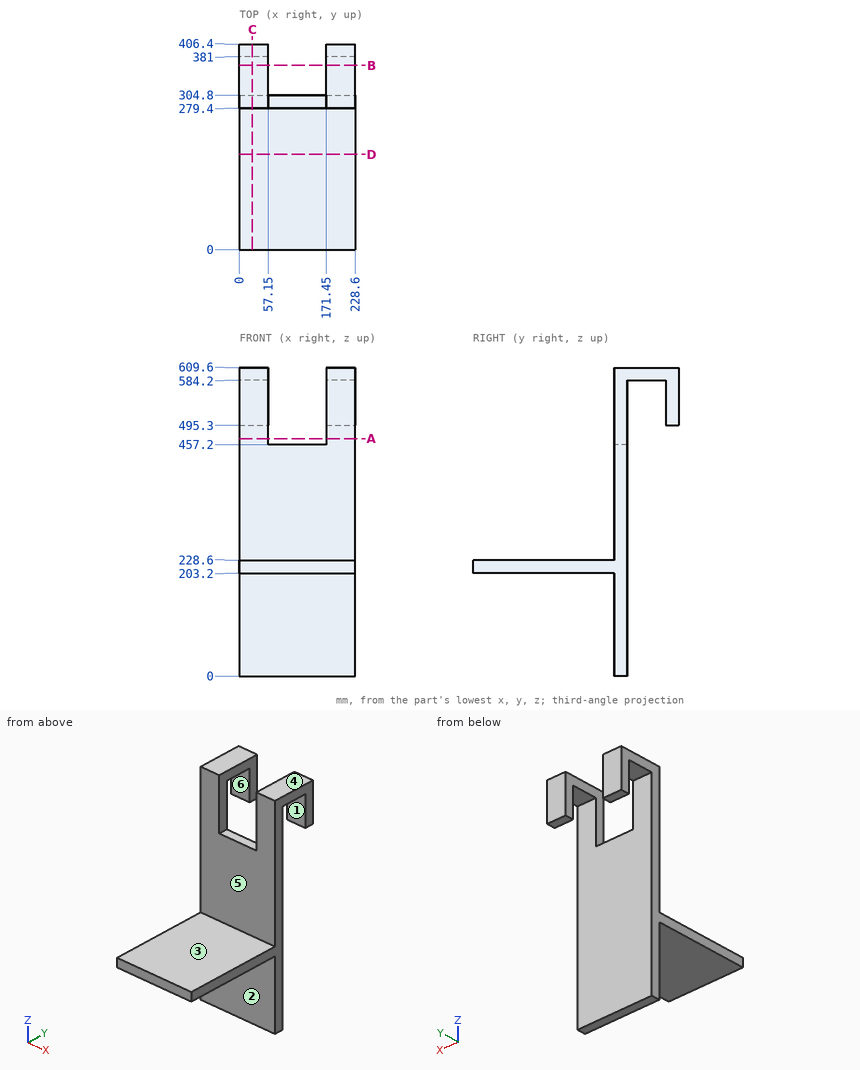
Geometry: see drawing. Coordinates: mm, zero at the bounding-box minimum. A direction names the side the tool comes from. Give positions to 0.01 mm unless a question says otherwise; leave off trailing zeros. Loops run counter-clockwise (first coordinate to the right, second up) from the corner with the lowest first, then second, coordinate; pieces in that order, holes last. Notation, with made-up numbers: (29.5, 61) - (46.5, 61) arc R19 cw to (46.5, 74) - close; hole circle Ø1 at (-11, 69). An arc over 180 degrees is marked (long way). Use CSV: the item, a comma, the result in double quotes. Start each with the question number.
1. Section B-B (y = 364). Output: boundary loops of the cut face in (x, z).
2. Reachability of the marked faces 1, 2 and 3 from +Z, -Z, +X, -X, +Y, -Y: full face, straight path, thin tool, end or side. Return the list, or none.
3. Pin query (flat end, axial travel): pin 1 (2 mm diameter, centred on x = 182, z = 534, fed in from -Y); pin 2 (7.5 mm diameter, centred on x = 91, y = 297, fed in from +Z); pin 3 (1 mm diameter, centred on x = 53, y = 174.5, fed in from -Z). Return the tip coordinate at first contact, or that it passes through.
4. Section C-C (x = 25.5). Output: boundary loops of the cut face in (y, z), then the cut area to 3 significant figures.
5. Section D-D (y = 188). Output: boundary loops of the cut face in (x, z), then the cut area to 3 significant figures.
6. Section A-A (z = 469). Output: boundary loops of the cut face in (x, y), then the cut area to 3 significant figures.
7. Draft query along Y for the marked faces 4, 5 and 6. Return one class per face: +Y half, -Y half, draft (parallel to the pull), parting line (faces both ways), or undercut.
8. Ray query, L1, parallel to X at y = 304.5, z = 529.5; L2, parallel to Y at x = 173, z = 519.5; L3, parallel to Z at x = 141, y = 169.5. Return the intervals inside material, ascending.
Response:
1,outline,"(0, 584.2) - (57.15, 584.2) - (57.15, 609.6) - (0, 609.6) - close; (171.45, 584.2) - (228.6, 584.2) - (228.6, 609.6) - (171.45, 609.6) - close"
2,face 1,"-Z, +X, -X"
2,face 2,"-Z, +X, -X, -Y"
2,face 3,"+Z, +X, -X, -Y"
3,pin 1,"y = 279.4"
3,pin 2,"z = 457.2"
3,pin 3,"z = 203.2"
4,outline,"(0, 203.2) - (279.4, 203.2) - (279.4, 0) - (304.8, 0) - (304.8, 584.2) - (381, 584.2) - (381, 495.3) - (406.4, 495.3) - (406.4, 609.6) - (279.4, 609.6) - (279.4, 228.6) - (0, 228.6) - close"
4,area,"27,400 mm²"
5,outline,"(0, 203.2) - (228.6, 203.2) - (228.6, 228.6) - (0, 228.6) - close"
5,area,"5,810 mm²"
6,outline,"(0, 279.4) - (57.15, 279.4) - (57.15, 304.8) - (0, 304.8) - close; (171.45, 279.4) - (228.6, 279.4) - (228.6, 304.8) - (171.45, 304.8) - close"
6,area,"2,900 mm²"
7,face 4,"draft"
7,face 5,"-Y half"
7,face 6,"undercut"
8,L1,"0 to 57.15, 171.45 to 228.6"
8,L2,"279.4 to 304.8, 381 to 406.4"
8,L3,"203.2 to 228.6"
